Autodesk Inventor part; units mm, degrees
ref_plane "YZ Plane" through (0, 0, 0) normal (1, 0, 0) x (0, 1, 0)
ref_plane "XZ Plane" through (0, 0, 0) normal (0, 1, 0) x (-1, 0, 0)
ref_plane "XY Plane" through (0, 0, 0) normal (0, 0, 1) x (1, 0, 0)
sketch "Sketch3" plane through (0, 0, 0) normal (0, 1, 0) x (-1, 0, 0)
  line L0 (50, 50) -> (-50, 50)
  line L1 (-50, 50) -> (-50, -50)
  line L2 (-50, -50) -> (50, -50)
  line L3 (50, -50) -> (50, 50)
  line L4 (50, 50) -> (-50, -50) construction
  line L5 (-50, 50) -> (50, -50) construction
  line L6 (45, -45) -> (-45, 45) construction
  line L7 (-45, -45) -> (45, 45) construction
  point P0 (0, 0)
  dimension "d12" = 100
  dimension "d13" = 100
extrude "Solid Mass" add sketch "Sketch3" along normal blind 40
sketch "Sketch6" plane through (50, 0, 50) normal (1, 0, 0) x (0, 0, -1)
  line L0 (0, 0) -> (100, 0)
  line L1 (0, 0) -> (10, 5)
  line L2 (10, 5) -> (15, 40)
  line L3 (0, 40) -> (100, 40)
  line L4 (0, 0) -> (0, 40)
  line L5 (100, 40) -> (25, 40)
  line L6 (25, 40) -> (25, 10)
  line L7 (25, 10) -> (100, 10)
  line L8 (100, 10) -> (100, 40)
  circle A0 centre (69.125, 22) radius 22.5
  line L9 (63.125, 17) -> (75.125, 17)
  line L10 (75.125, 17) -> (75.125, 27)
  line L11 (75.125, 27) -> (63.125, 27)
  line L12 (63.125, 27) -> (63.125, 17)
  line L13 (63.125, 17) -> (75.125, 27) construction
  line L14 (75.125, 17) -> (63.125, 27) construction
  line L15 (100, 0) -> (100, 40)
  line L16 (52.125, 10) -> (52.125, 17)
  line L17 (55.125, 10) -> (55.125, 14)
  line L18 (55.125, 14) -> (63.125, 14)
  line L19 (63.125, 14) -> (63.125, 10)
  line L20 (69.125, 22) -> (69.125, 0)
  line L21 (52.125, 17) -> (69.125, 17)
  line L22 (86.125, 10) -> (86.125, 17)
  line L23 (83.125, 10) -> (83.125, 14)
  line L24 (83.125, 14) -> (75.125, 14)
  line L25 (75.125, 14) -> (75.125, 10)
  line L26 (86.125, 17) -> (69.125, 17)
  point P0 (50, 0)
  point P1 (25, 40)
  point P2 (82.625, 40)
  point P3 (88.1579, 10)
  point P4 (64.408, 0)
  point P5 (50.0921, 10)
  point P6 (67.25, 14)
  point P7 (55.625, 40)
  point P8 (55.25, 14)
  point P9 (73.842, 0)
  point P10 (75.125, 10)
  point P11 (83.125, 10)
  point P12 (86.125, 10)
  point P13 (75.125, 17)
  dimension "d20" = 10
  dimension "d21" = 5
  dimension "d22" = 15
  dimension "d25" = 10
  dimension "d27" = 45
  dimension "d28" = 12
  dimension "d29" = 10
  dimension "d35" = 15
  dimension "d45" = 22
  dimension "d47" = 30.875
  dimension "d48" = 3
  dimension "d49" = 3
  dimension "d50" = 11
extrude "Cut Ramp" cut sketch "Sketch6" against normal through all contours L4 L3 L2 L1 | A0 L3 L7 L22 L26 L10 L11 L12 L21 L16 | L7 L6 L3 A0 | L20 L9 L26 L22 L7 L23 L24 L25 | L7 L19 L18 L17 L16 L21 L9 L20 | A0 L3 L8 L7 | L7 L17 L18 L19 | L25 L24 L23 L7 | L9 L12 L11 L10
sketch "Sketch7" plane through (50, 10, 25) normal (0, 0, -1) x (-1, 0, 0)
  circle A0 centre (62.75, 11) radius 8.5
  line L0 (100, 0) -> (0, 0)
  line L1 (0, 30) -> (100, 30)
  line L2 (0, 0) -> (0, 30)
  line L3 (0, -10) -> (0, 0)
  line L4 (100, -10) -> (100, 0)
  line L5 (100, 30) -> (100, 0)
  line L6 (0, -10) -> (100, -10)
  line L7 (50, 30) -> (50, 0)
  circle A1 centre (37.25, 11) radius 8.5
  line L8 (58.2723, 18.225) -> (62.75, 21)
  line L9 (62.75, 21) -> (67.2277, 18.225)
  line L10 (41.7277, 18.225) -> (37.25, 21)
  line L11 (37.25, 21) -> (32.7723, 18.225)
  point P0 (50, -10)
  point P1 (32.7723, 18.225)
  point P2 (41.7277, 18.225)
  dimension "d30" = 17
  dimension "d31" = 11
  dimension "d32" = 25.5
  dimension "d46" = 10
extrude "Eyes" cut sketch "Sketch7" against normal through all contours A0 | A0 L8 L9 | A1 | A1 L11 L10
extrude "Motor Platform" add sketch "Sketch6" against normal up to surface (100 mm away) contours L20 L9 L26 L22 L7 L23 L24 L25 | L7 L19 L18 L17 L16 L21 L9 L20
sketch "Sketch9" plane through (-50, 0, -50) normal (-1, 0, 0) x (0, 0, 1)
  line L0 (5, 22) -> (5, 0)
  line L1 (56.75, 22) -> (56.75, 0)
  arc A0 (56.75, 22) -> (5, 22) centre (30.875, 22) ccw
  line L2 (5, 0) -> (56.75, 0)
  line L3 (0, 10) -> (13.875, 10)
  line L4 (24.875, 17) -> (24.875, 27)
  line L5 (24.875, 27) -> (36.875, 27)
  line L6 (36.875, 27) -> (36.875, 17)
  line L7 (13.875, 17) -> (47.875, 17)
  line L8 (13.875, 10) -> (0, 10)
  circle A1 centre (30.875, 22) radius 22.5
  line L9 (0, 0) -> (100, 0)
  line L10 (0, 0) -> (0, 10)
  point P0 (50, 0)
  point P1 (5, 10)
  point P2 (26.158, 0)
  point P3 (11.8421, 10)
  point P4 (35.592, 0)
  dimension "d54" = 5
  dimension "d55" = 51.75
  dimension "d56" = 22
extrude "Cut right wheel" cut sketch "Sketch9" against normal blind 20 contours A0 L1 L2 A1 L3 L0 | L3 A1 L2 L0 | A1 L2 | L4 L5 L6 L7 picked at (31.5427, 32.8036)
extrude "Cut left wheel" cut sketch "Sketch9" along normal blind 20 from surface at -100 contours A0 L1 L2 A1 L3 L0 | L3 A1 L2 L0 | A1 L2 | L4 L5 L6 L7 picked at (31.5427, 32.8036)
sketch "Sketch8" plane through (50, 10, 25) normal (0, 1, 0) x (1, 0, 0)
  line L0 (-27, 35) -> (-27, 36) construction
  line L1 (-25.75, 35) -> (-25.75, 36)
  line L2 (-28.25, 36) -> (-28.25, 35)
  arc A0 (-28.25, 35) -> (-25.75, 35) centre (-27, 35) ccw
  arc A1 (-25.75, 36) -> (-28.25, 36) centre (-27, 36) ccw
  line L3 (-27, 52.5) -> (-27, 53.5) construction
  line L4 (-25.75, 52.5) -> (-25.75, 53.5)
  line L5 (-28.25, 53.5) -> (-28.25, 52.5)
  arc A2 (-28.25, 52.5) -> (-25.75, 52.5) centre (-27, 52.5) ccw
  arc A3 (-25.75, 53.5) -> (-28.25, 53.5) centre (-27, 53.5) ccw
  line L6 (-100, 0) -> (-100, 18.25)
  line L7 (0, 0) -> (-100, 0)
  line L8 (0, 75) -> (0, 70)
  line L9 (-100, 75) -> (0, 75)
  line L10 (-100, 75) -> (0, 75)
  line L11 (-50, 75) -> (-50, 0)
  line L12 (-73, 35) -> (-73, 36) construction
  line L13 (-74.25, 35) -> (-74.25, 36)
  line L14 (-71.75, 36) -> (-71.75, 35)
  arc A4 (-74.25, 35) -> (-71.75, 35) centre (-73, 35) ccw
  arc A5 (-71.75, 36) -> (-74.25, 36) centre (-73, 36) ccw
  line L15 (-73, 52.5) -> (-73, 53.5) construction
  line L16 (-74.25, 52.5) -> (-74.25, 53.5)
  line L17 (-71.75, 53.5) -> (-71.75, 52.5)
  arc A6 (-74.25, 52.5) -> (-71.75, 52.5) centre (-73, 52.5) ccw
  arc A7 (-71.75, 53.5) -> (-74.25, 53.5) centre (-73, 53.5) ccw
  line L18 (0, 0) -> (-100, 0)
  line L19 (-27, 0) -> (-27, 75) construction
  line L20 (-80, 18.25) -> (-100, 18.25)
  line L21 (0, 18.25) -> (0, 0)
  line L22 (0, 18.25) -> (-20, 18.25)
  line L23 (-20, 27.125) -> (-20, 18.25)
  line L24 (-20, 27.125) -> (-80, 27.125)
  line L25 (-80, 27.125) -> (-80, 18.25)
  line L26 (-100, 70) -> (-100, 75)
  line L27 (-100, 70) -> (-80, 70)
  line L28 (-80, 70) -> (-80, 61.125)
  line L29 (-80, 61.125) -> (-20, 61.125)
  line L30 (-20, 70) -> (-20, 61.125)
  line L31 (-20, 70) -> (0, 70)
  point P0 (-50, 25)
  point P1 (-27, 35.5)
  point P2 (-27, 53)
  point P3 (-73, 35.5)
  point P4 (-73, 53)
  point P5 (-50, 61.125)
  point P6 (-50, 27.125)
  dimension "d36" = 17.5
  dimension "d37" = 1.25
  dimension "d38" = 1
  dimension "d40" = 27
  dimension "d41" = 22
extrude "Cut Motor Bolt Holes" cut sketch "Sketch8" along normal blind 20 contours A0 L2 A1 L1 | A2 L5 A3 L4 | L13 A5 L14 A4 | L16 A7 L17 A6
sketch "Sketch10" plane through (-30, 10, -36.125) normal (0, 0, -1) x (-1, 0, 0)
  line L0 (-60, 0) -> (-60, 7)
  line L1 (-60, 7) -> (0, 7)
  line L2 (0, 0) -> (0, 7)
  line L3 (0, 0) -> (-60, 0)
  line L4 (-46, 7) -> (-14, 7)
  line L5 (-14, 7) -> (-14, 0)
  line L6 (-14, 0) -> (-46, 0)
  line L7 (-46, 0) -> (-46, 7)
  point P0 (-30, -10)
  point P1 (-46, 0)
  dimension "d61" = 14
  dimension "d62" = 14
extrude "Cut Centre" cut sketch "Sketch10" against normal up to surface (34 mm away) contours L7 L1 L5 L3
sketch "Sketch12" plane through (0, 0, 0) normal (0, -1, 0) x (1, 0, 0)
  line L0 (50, 25) -> (-50, 25)
  line L1 (-21.5, 18) -> (21.5, 18)
  line L2 (21.5, 18) -> (21.5, 6)
  line L3 (21.5, 6) -> (-21.5, 6)
  line L4 (-21.5, 6) -> (-21.5, 18)
  point P0 (0, 0)
  point P1 (0, 6)
  dimension "d72" = 43
  dimension "d73" = 12
  dimension "d74" = 7
extrude "Extrusion13" cut sketch "Sketch12" against normal blind 10
sketch "Sketch13" plane through (50, 10, 25) normal (0, 0, -1) x (-1, 0, 0)
  line L0 (27.25, 21) -> (72.75, 21)
  line L1 (72.75, 21) -> (72.75, 1)
  line L2 (72.75, 1) -> (27.25, 1)
  line L3 (27.25, 1) -> (27.25, 21)
  arc A0 (58.2723, 18.225) -> (67.2277, 18.225) centre (62.75, 11) ccw
  circle A1 centre (62.75, 11) radius 10 construction
  arc A2 (32.7723, 18.225) -> (41.7277, 18.225) centre (37.25, 11) ccw
  circle A3 centre (37.25, 11) radius 10 construction
  line L4 (44, 5.5) -> (56, 5.5)
  line L5 (56, 5.5) -> (56, 1.5)
  line L6 (56, 1.5) -> (44, 1.5)
  line L7 (44, 1.5) -> (44, 5.5)
  circle A4 centre (54, 3.5) radius 2
  circle A5 centre (46, 3.5) radius 2
  line L8 (45, 20.5) -> (55, 20.5)
  line L9 (55, 20.5) -> (55, 17.5)
  line L10 (55, 17.5) -> (45, 17.5)
  line L11 (45, 17.5) -> (45, 20.5)
  point P0 (50, -10)
  point P1 (50, 5.5)
  point P2 (50, 1)
  point P3 (50, 20.5)
  point P4 (50, 21)
  point P5 (46, 1.5)
  point P6 (54, 1.5)
  point P7 (54, 5.5)
  point P8 (46, 5.5)
  dimension "d75" = 20
  dimension "d76" = 20
  dimension "d77" = 20
  dimension "d78" = 12
  dimension "d79" = 4
  dimension "d80" = 0.5
  dimension "d81" = 10
  dimension "d82" = 3
  dimension "d83" = 0.5
extrude "Extrusion14" cut sketch "Sketch13" against normal blind 5 contours L4 A4 L6 A5 | A5 | A4 | L8 L9 L10 L11
sketch "Sketch16" plane through (-21.5, 0, 18) normal (1, 0, 0) x (0, 0, -1)
  line L0 (12, 0) -> (12, 10)
  line L1 (0, 0) -> (0, 10)
  line L2 (12, 0) -> (0, 0)
  line L3 (0, 0) -> (0, 4)
  line L4 (0, 4) -> (12, 4)
  line L5 (12, 4) -> (12, 0)
  point P0 (18, 0)
  dimension "d89" = 4
extrude "Extrusion16" cut sketch "Sketch16" against normal blind 34
sketch "Sketch17" plane through (-50, 10, 25) normal (0, 1, 0) x (1, 0, 0)
  line L0 (20, 18.25) -> (0, 18.25)
  line L1 (0, 7) -> (71.5, 7)
  line L2 (0, 18.25) -> (10, 18.25)
  line L3 (10, 18.25) -> (10, 7)
  line L4 (10, 7) -> (0, 7)
  line L5 (0, 7) -> (0, 18.25)
  point P0 (50, 25)
  dimension "d92" = 10
extrude "Extrusion17" cut sketch "Sketch17" against normal blind 34
sketch "Sketch18" plane through (-50, 10, 25) normal (0, 1, 0) x (1, 0, 0)
  line L0 (71.5, 7) -> (28.5, 7)
  line L1 (71.5, 19) -> (71.5, 7)
  line L2 (28.5, 19) -> (71.5, 19)
  line L3 (28.5, 7) -> (28.5, 19)
  line L4 (27.5, 6) -> (72.5, 6)
  line L5 (72.5, 6) -> (72.5, 20)
  line L6 (72.5, 20) -> (27.5, 20)
  line L7 (27.5, 20) -> (27.5, 6)
  point P0 (50, 25)
  dimension "d95" = 1
extrude "Extrusion18" add sketch "Sketch18" along normal blind 3
sketch "Sketch19" plane through (-50, 13, 25) normal (0, 1, 0) x (1, 0, 0)
  line L0 (28.5, 7) -> (28.5, 19)
  line L1 (71.5, 7) -> (28.5, 7)
  line L2 (28.5, 7) -> (28.5, 19)
  line L3 (28.5, 19) -> (71.5, 19)
  line L4 (71.5, 19) -> (71.5, 7)
  point P0 (50, 25)
  point P1 (28.5, 7)
extrude "Extrusion19" add sketch "Sketch19" against normal blind 1.5
sketch "Sketch20" plane through (-30, 0, -50) normal (-1, 0, 0) x (0, 0, 1)
  line L0 (24.875, 14) -> (16.875, 14)
  line L1 (36.875, 10) -> (44.875, 10)
  line L2 (24.875, 14) -> (36.875, 14)
  line L3 (36.875, 14) -> (36.875, 10)
  line L4 (36.875, 10) -> (24.875, 10)
  line L5 (24.875, 10) -> (24.875, 14)
  point P0 (50, 0)
extrude "Extrusion20" cut sketch "Sketch20" against normal blind 100
fillet "Fillet1" radius 3 1 edges at (0, 13, 19)
sketch "Sketch21" plane through (-50, 10, -50) normal (0, 1, 0) x (1, 0, 0)
  line L0 (59.9918, -13.8859) -> (42.201, -13.8859)
  line L1 (42.201, -13.8859) -> (42.201, -46.4739)
  line L2 (42.201, -46.4739) -> (59.9918, -46.4739)
  line L3 (59.9918, -46.4739) -> (59.9918, -13.8859)
  point P0 (50, -50)
properties part number "shell_01"
Work out the finished part from the listing and answer in its coordinate system (mm). A direction names the side the tool comes from. Coordinates: 2 decimals unless noted, no trailing zeros. Loops run counter-clockwise (first coordinate to the right, second up) from the corner with the lowest first, then second, coordinate; pieces in that order, holes last. Notation, with made-up numbers: (35.5, 23.25) - (62.5, 23.25) arc R30 ccw to (62.5, 53.25) - close; hole circle Ø9 at (-1.75, 74). An arc over 180 degrees is marked (long way). Use a Markdown table: item, result.
Item 1: Given pin 1 Ø5 at (x, y) = (40, 31.5) entering from -Z; pin 2 Ø2 at (x, y) = (23.5, 12.5) entering from -Z (3 decimals); pin 3 Ø19.5 at (x, y) = (-12.75, 21) entering from +Z, each flat-ended and moving along its own axis, determine where each tip first touches the part or whether it passes through.
Evaluation:
| item | result |
|---|---|
| pin 1 | stops at z = 25 |
| pin 2 | stops at z = -36.125 |
| pin 3 | stops at z = 39.11 |
Item 2: The mould has two halves that part along Z. Classify faces 6 (the flat face through (23, 14, -19)), 7 (the flat face through (0, 27.5, 27)): +Z half, -Z half, draft (parallel to the pull), parting line (faces both ways), or undercut.
Evaluation:
| item | result |
|---|---|
| face 6 | undercut |
| face 7 | draft |
Item 3: Find section C-C, the plane x = 43.5. Determine the outline of the cut face in (y, z), and give its area (3 significant figures).
Evaluation:
| item | result |
|---|---|
| outline | (0, -50) - (10, -50) - (10, -45) - (0, -45) - close; (0, 6.75) - (10, 6.75) - (10, 25) - (40, 25) - (40, 35) - (5, 40) - (0, 50) - close |
| area | 770 mm2 |
Item 4: Find section A-A, the plane x = -36.5. Determine the outline of the cut face in (y, z), and give its area (3 significant figures).
Evaluation:
| item | result |
|---|---|
| outline | (0, -50) - (10, -50) - (10, -45) - (0, -45) - close; (0, 18) - (4, 18) - (4, 6.75) - (10, 6.75) - (10, 25) - (40, 25) - (40, 35) - (5, 40) - (0, 50) - close |
| area | 725 mm2 |
Item 5: Find section B-B, the plane y = 19.5. Determine the outline of the cut face in (x, z), and give its area (3 significant figures).
Evaluation:
| item | result |
|---|---|
| outline | (-50, 25) - (-21.12, 25) - (-21.12, 37.93) - (-50, 37.93) - close; (-4.38, 25) - (4.38, 25) - (4.38, 37.93) - (-4.38, 37.93) - close; (21.12, 25) - (50, 25) - (50, 37.93) - (21.12, 37.93) - close |
| area | 860 mm2 |
Item 6: Consider probe 1 along X at (y, z) = (21, 32); probe 2 along Y at (x, z) = (12.75, 29.5); probe 3 along X at (y, z) = (28.5, 29). Determine where each line is inside the solid, lowest interval first. Write a range as from..to.
Evaluation:
| item | result |
|---|---|
| probe 1 | x = -50..-21.25, -4.25..4.25, 21.25..50 |
| probe 2 | y = 0..12.5, 31..40 |
| probe 3 | x = -50..-16.78, -8.72..-5, 5..8.72, 16.78..50 |
Item 7: For faces 1 (the flat face through (-5, 29, 27)), 2 (the cylindrical face through (-22.97, 15.48, -26.25)), 3 (the flat face through (-10.48, 29.593, 30.759)), 4 (the flat face through (-31, 4, 12)), 5 (the cylindrical face through (6, 13.5, 27.5)), determine the directions among +Z, -Z, +X, -X, +Y, -Y from which every point of the face is accessible in a straight line to the end or side of a thin tool.
Evaluation:
| item | result |
|---|---|
| face 1 | -Z |
| face 2 | +Y |
| face 3 | +Z, -Z |
| face 4 | -X, -Y |
| face 5 | none |
